Geometry: final body of the model. Coordinates: model frame, mm. A direction names the side the tool comes from. Coordinates: 2 decimals unless noted, no trailing zeros. Loops run counter-clockwise (first coordinate to the right, second up) from the corner with the lowest first, then second, coordinate; pieces in that order, holes last. Notation, with made-up numbers: (-14, 78) - (30, 78) arc R15 ccw to (30, 84) - close; hole circle Ø6 at (46, 61). An arc over 180 degrees is marked (long way). Answer in a Markdown table with one row per item.
from build123d import *

# Parameters (mm, degrees)
F0_W     = 330.2
F0_H     = 317.5
F1_DEPTH = 3.175
F2_W     = 330.2
F2_H     = 3.175
F3_DEPTH = 190.5
F4_W     = 330.2
F4_H     = 190.5
F5_DEPTH = 25.4


with BuildPart() as f1:
    # F0 (on Front) → F1 (new body)
    with BuildSketch(Plane.XZ):
        with Locations((165.1, 158.75)):
            Rectangle(F0_W, F0_H)
    extrude(amount=F1_DEPTH)

    # F2 (on face) → F3 (join)
    with BuildSketch(Plane.XY.offset(317.5)):
        with Locations((165.1, -1.5875)):
            Rectangle(F2_W, F2_H)
    extrude(amount=F3_DEPTH)

    # F4 (on face) → F5 (join)
    with BuildSketch(Plane.XZ.offset(3.175)):
        with Locations((165.1, 412.75)):
            Rectangle(F4_W, F4_H)
    extrude(amount=F5_DEPTH)


solid = f1.part
(1) Ray query, probe 1 along Y at (x, z) = (45.5, 50.5) (3 decimals); probe 2 along Z at (x, y) = (96, -7.75). Return the intervals inside material, ascending.
Verdict:
| item | result |
|---|---|
| probe 1 | y = -3.175 to 0 |
| probe 2 | z = 317.5 to 508 |
(2) Access query for faces 1 (the face through (163, -16, 317.5)), 2 (the face through (330.2, -11, 363)). Directions: +Z, -Z, +X, -X, +Y, -Y. A direction counts if a zero-diameter tool reaches every point of the face in a straight line with its end or side. Return the directions, or none.
Verdict:
| item | result |
|---|---|
| face 1 | -Z, +X, -X, -Y |
| face 2 | +Z, -Z, +X, +Y, -Y |
(3) Cut plane C-C on z = 115.5. Output: boundary loops of the cut face in (x, y) (3 decimals), then the cut area to 3 significant figures.
Verdict:
| item | result |
|---|---|
| outline | (0, -3.175) - (330.2, -3.175) - (330.2, 0) - (0, 0) - close |
| area | 1,050 mm² |
(4) Cut plane A-A on x = 296. Output: boundary loops of the cut face in (y, z) (3 decimals), then the cut area to 3 significant figures.
Verdict:
| item | result |
|---|---|
| outline | (-28.575, 317.5) - (-3.175, 317.5) - (-3.175, 0) - (0, 0) - (0, 508) - (-28.575, 508) - close |
| area | 6,450 mm² |
(5) Cut plane B-B on y = -24. Output: boundary loops of the cut face in (x, z), then the cut area to 3 significant figures.
Verdict:
| item | result |
|---|---|
| outline | (0, 317.5) - (330.2, 317.5) - (330.2, 508) - (0, 508) - close |
| area | 62,900 mm² |
(6) First-contact query: pin 1 Ø3 at (x, y) = (112.5, -19.5) entering from -Z; pin 2 Ø1.5 at (x, z) = (102.5, 115) entering from -Y (3 decimals). Flat tips, straight axial feed; report the tip coordinate or a pass-through.
Verdict:
| item | result |
|---|---|
| pin 1 | stops at z = 317.5 |
| pin 2 | stops at y = -3.175 |
